Study the drawing (mm; zero at the part's minimum x, y, z) and answer. Coordinates: 2 decimals unless noted, no trailing zeros. Loops run counter-clockwise (first coordinate to the right, second up) from the corner with the lowest first, then second, coordinate; pieces in that order, holes last. Notation, with made-up numbers: (16.5, 58) - (65.5, 58) arc R13 cw to (65.5, 80) - close; hole circle Ø8 at (36, 60). An arc over 180 degrees is marked (long way). Write each question's results on one line, items separated by ' | '. Start each with the question number.
(1) Find section D-D on x = 16.75. Determine the outline of the cut face in (y, z), then the cut area to 3 significant figures.
(2) Given pin 1 Ø8 at (x, y) = (12.5, 12.5) entering from +Z; pin 2 Ø10 at (y, z) = (3.5, 6) entering from +X; pin 3 Ø6 at (x, z) = (20.5, 35) entering from -Y, each flat-ended and moving along its own axis, determine where each tip first touches the part or whether it passes through.
(3) Determine the mould class of the marked faces 1, 2 and 3 for opening direction X: released by +X, released by -X, zero draft, split by the parting line, or undercut.
(4) Consider line 1 (Y direction, x = 12.5, z = 21.5); line 2 (Z direction, x = 12.5, y = 7.25); line 3 (Y direction, x = 12.5, z = 4.75). Determine where each line is inside the solid, lowest interval first. Write a range as from..to.
(5) Find section C-C on z = 11. Determine the outline of the cut face in (x, y), then the cut area to 3 significant figures.
(6) Find section B-B on y = 15.5. Determine the outline of the cut face in (x, z).
(7) Find section A-A on x = 12.5. Determine the outline of the cut face in (y, z), then the cut area to 4 significant figures.
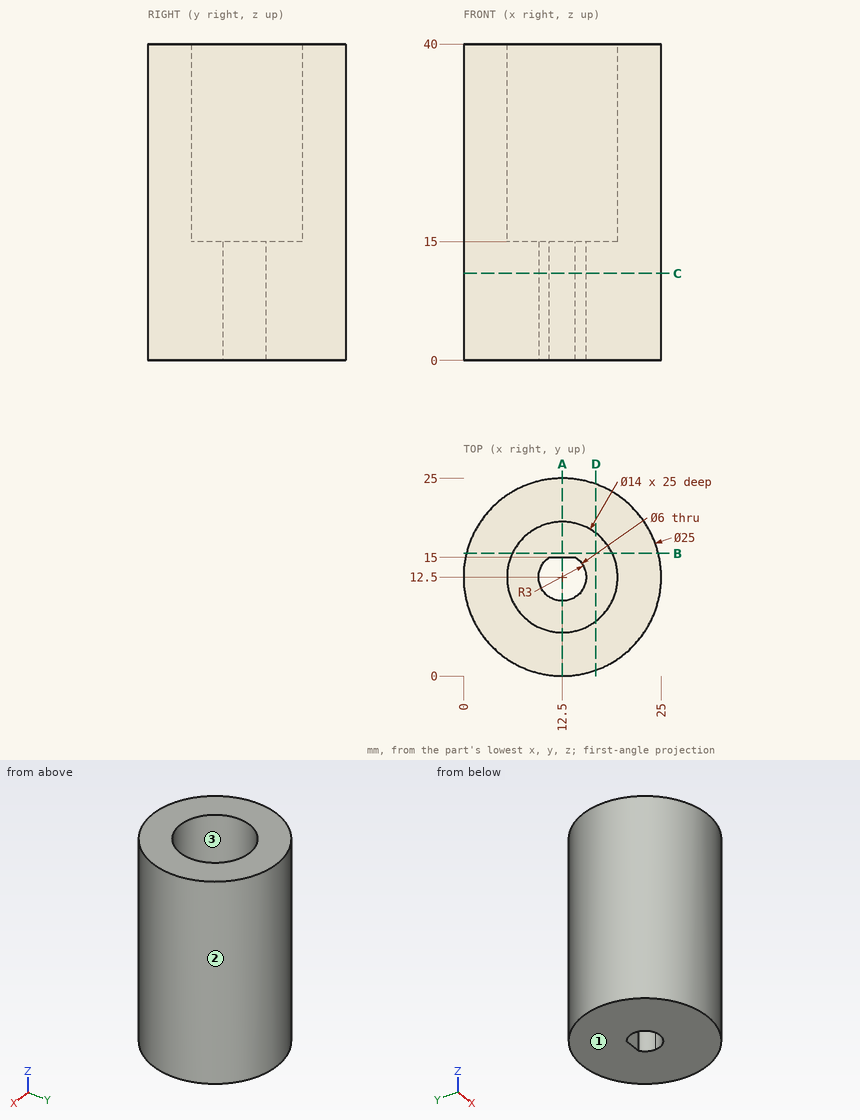
Values:
1) outline: (0.74, 0) - (24.26, 0) - (24.26, 40) - (18.06, 40) - (18.06, 15) - (6.94, 15) - (6.94, 40) - (0.74, 40) - close | area: 662 mm²
2) pin 1: stops at z = 15 | pin 2: stops at x = 24.34 | pin 3: stops at y = 1.04
3) face 1: zero draft | face 2: split by the parting line | face 3: undercut
4) line 1: y = 0..5.5, 19.5..25 | line 2: z = 0..15 | line 3: y = 0..9.5, 15..25
5) outline: circle Ø25 at (12.5, 12.5); hole (10.84, 15) arc R3 ccw (long way) to (14.16, 15) - close | area: 464 mm²
6) outline: (0.37, 0) - (24.63, 0) - (24.63, 40) - (18.82, 40) - (18.82, 15) - (6.18, 15) - (6.18, 40) - (0.37, 40) - close
7) outline: (0, 0) - (9.5, 0) - (9.5, 15) - (5.5, 15) - (5.5, 40) - (0, 40) - close; (15, 0) - (25, 0) - (25, 40) - (19.5, 40) - (19.5, 15) - (15, 15) - close | area: 567.5 mm²
